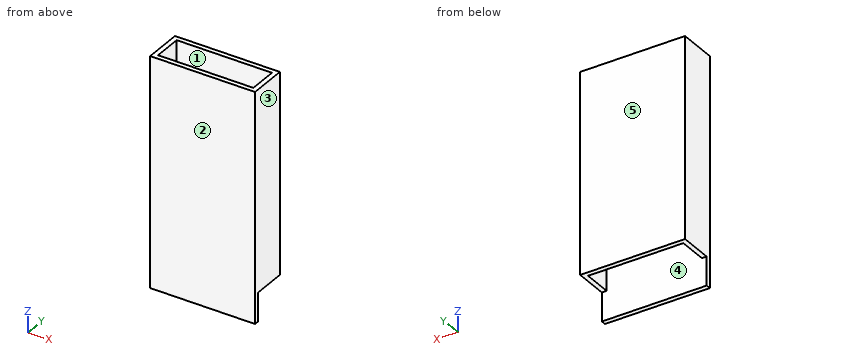
from build123d import *

# Parameters (mm, degrees)
SKETCH1_W           = 220
SKETCH1_H           = 80
SKETCH1_W_2         = 200
SKETCH1_H_2         = 60
BOSS_EXTRUDE1_DEPTH = 420
SKETCH3_W           = 220
SKETCH3_H           = 10
BOSS_EXTRUDE3_DEPTH = 60


with BuildPart() as part:
    # Sketch1 → Boss-Extrude1 (new body)
    with BuildSketch(Plane.XY):
        Rectangle(SKETCH1_W, SKETCH1_H)
        Rectangle(SKETCH1_W_2, SKETCH1_H_2, mode=Mode.SUBTRACT)
    extrude(amount=BOSS_EXTRUDE1_DEPTH)

    # Sketch3 → Boss-Extrude3 (add)
    with BuildSketch(Plane(origin=(0, 0, 0), x_dir=(-1, 0, 0), z_dir=(0, 0, -1))):
        with Locations((0, -35)):
            Rectangle(SKETCH3_W, SKETCH3_H)
    extrude(amount=BOSS_EXTRUDE3_DEPTH)


solid = part.part
Model file for the job. Use its own axes, mm. Face numbers are marked on the shaded views. A direction names the side the tool comes from. Give positions to 0.01 mm unless a question says otherwise; leave off trailing zeros. Order: outer loops, then holes, each group sorted by start corner. A loop starts at its lowest first (then second) coordinate and runs counter-clockwise, first axis right, second up. Notation, with made-up numbers: (-26, -22) -> (4, -22) arc R23 ccw to (4, -13) -> close; hole circle Ø2 at (32.25, 40). An arc over 180 degrees is marked (long way). Use CSV: the item, a comma, the result in double quotes.
1. Mould opens along Y. For the marked faces 3, 4 and 5 say: +Y half, -Y half, draft (parallel to the pull), parting line (faces both ways), or undercut.
Outcome:
face 3,"draft"
face 4,"undercut"
face 5,"+Y half"
2. Band-saw the part on B-B, the plane z = 305. Give the cut face in (x, y).
Outcome:
outline,"(-110, -40) -> (110, -40) -> (110, 40) -> (-110, 40) -> close; hole (-100, -30) -> (100, -30) -> (100, 30) -> (-100, 30) -> close"
3. Band-saw the part on C-C, the plane x = 71. Give the cut face in (y, z), then the cut area to 3 significant figures.
Outcome:
outline,"(-40, -60) -> (-30, -60) -> (-30, 420) -> (-40, 420) -> close; (30, 0) -> (40, 0) -> (40, 420) -> (30, 420) -> close"
area,"9,000 mm²"
4. 3-axis set-ups, long thin cutter, end or side, ignore diameter. For the marked faces 1 and 2: which of +Z, -Z, +X, -X, +Y, -Y reach the whole face in a straight line?
Outcome:
face 1,"+Z, -Z"
face 2,"+Z, -Z, +X, -X, -Y"
5. Band-saw the part on A-A, the plane y = -16. Give the cut face in (x, z).
Outcome:
outline,"(-110, 0) -> (-100, 0) -> (-100, 420) -> (-110, 420) -> close; (100, 0) -> (110, 0) -> (110, 420) -> (100, 420) -> close"
6. Drill centre lines: line 1 along Y through (x, z) = (-8, 389); line 2 along X through (y, z) = (-13, 154); line 3 along Z through (x, y) = (-92, 37). Where is each one in solid material? Low to high. Write a range as from..to.
Outcome:
line 1,"-40..-30, 30..40"
line 2,"-110..-100, 100..110"
line 3,"0..420"
